The listing builds one solid part. Answer for the finished solid, in the listing's coordinates (mm). A direction names the side the tool comes from. Give positions to 0.01 mm unless a question says otherwise; leave off trailing zeros. Order: outer loops, then holes, each group sorted by start corner. A loop starts at its lowest first (then second) coordinate and runs counter-clockwise, first axis right, second up. Notation, with made-up numbers: (48, 12.25) - (93, 12.25) arc R21 ccw to (93, 39.25) - close; hole circle Ø1 at (17, -11). An arc over 180 degrees is marked (long way). Answer in a Markdown table with one row per item.
from build123d import *

# Parameters (mm, degrees)
F0_W     = 44.45
F0_H     = 21.082
F1_DEPTH = 0.2645833334
F2_W     = 0.3908552
F2_H     = 0.508
F3_DEPTH = 22.225


with BuildPart() as f1:
    # F0 (on Front) → F1 (new body)
    with BuildSketch(Plane.XZ):
        Rectangle(F0_W, F0_H)
    extrude(amount=F1_DEPTH)

    # F2 (on Right) → F3 (join, symmetric)
    with BuildSketch(Plane.YZ):
        with Locations((0.1954276, 10.033)):
            Rectangle(F2_W, F2_H)
    extrude(amount=F3_DEPTH, both=True)


solid = f1.part
Item 1: Consider line 1 (Y direction, x = -14.5, z = 4.5); line 2 (Z direction, x = 10.5, y = 0.25). Determine where each line is inside the solid, lowest interval first.
Answer block:
| item | result |
|---|---|
| line 1 | -0.26 to 0 |
| line 2 | 9.78 to 10.29 |
Item 2: Which of the six approach directions +Z, -Z, +X, -X, +Y, -Y give full straight-line access (tool end or side, diameter ignored) to faces 1 (the face through (0, -0.265, 0)), 2 (the face through (0, 0, 0))?
Answer block:
| item | result |
|---|---|
| face 1 | +Z, -Z, +X, -X, -Y |
| face 2 | -Z, +X, -X, +Y |
Item 3: This flat-tipped pin is pushed along its axis until it touches: P1, Ø6, axis at x = -5.5, z = 3, coming from the +Y side. Where does it stop, or does it pass through?
Answer block:
| item | result |
|---|---|
| P1 | y = 0 |
Item 4: Find section C-C on y = 0.15. Write down the section's boundary in (x, z) (3 decimals), then the cut area to 3 significant figures.
Answer block:
| item | result |
|---|---|
| outline | (-22.225, 9.779) - (22.225, 9.779) - (22.225, 10.287) - (-22.225, 10.287) - close |
| area | 22.6 mm² |
Item 5: Find section A-A on x = -4.5. Write down the section's boundary in (y, z), then the cut area to 3 significant figures.
Answer block:
| item | result |
|---|---|
| outline | (-0.26, -10.54) - (0, -10.54) - (0, 9.78) - (0.39, 9.78) - (0.39, 10.29) - (0, 10.29) - (0, 10.54) - (-0.26, 10.54) - close |
| area | 5.78 mm² |
Item 6: Find section B-B on z = 6.5. Write down the section's boundary in (x, y) (3 decimals), then the cut area to 3 significant figures.
Answer block:
| item | result |
|---|---|
| outline | (-22.225, -0.265) - (22.225, -0.265) - (22.225, 0) - (-22.225, 0) - close |
| area | 11.8 mm² |
